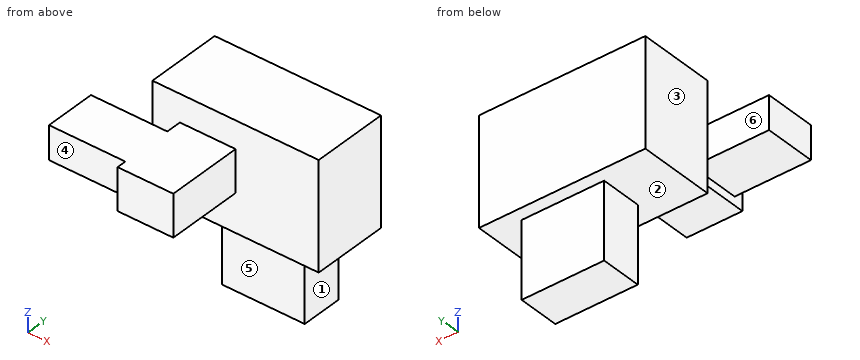
```python
from build123d import *

# Parameters (mm, degrees)
F0_W     = 55.336684
F0_H     = 35.7977
F1_DEPTH = 25.4
F2_W     = 18.540639
F2_H     = 13.976792
F3_DEPTH = 25.4
F4_W     = 17.11444
F4_H     = 11.124386
F5_DEPTH = 25.4
F6_W     = 27.447399
F6_H     = 13.715297
F7_DEPTH = 25.4


with BuildPart() as f1:
    # F0 (on Front) → F1 (new body)
    with BuildSketch(Plane.XZ):
        with Locations((27.668342, 17.89885)):
            Rectangle(F0_W, F0_H)
    extrude(amount=F1_DEPTH)

    # F2 (on face) → F3 (join)
    with BuildSketch(Plane.XZ.offset(25.4)):
        with Locations((18.39802, 19.681605)):
            Rectangle(F2_W, F2_H)
    extrude(amount=F3_DEPTH)

    # F4 (on face) → F5 (join)
    with BuildSketch(Plane(origin=(9.127701, 0, 0), x_dir=(0, -1, 0), z_dir=(-1, 0, 0))):
        with Locations((39.077966, 21.107808)):
            Rectangle(F4_W, F4_H)
    extrude(amount=F5_DEPTH)

    # F6 (on face) → F7 (join)
    with BuildSketch(Plane(origin=(0, 0, 0), x_dir=(1, 0, 0), z_dir=(0, 0, -1))):
        with Locations((30.881432, 11.093259)):
            Rectangle(F6_W, F6_H)
    extrude(amount=F7_DEPTH)


solid = f1.part
```
Build history of the part. All positions in model axes, mm. Face numbers are marked on the shaded views. A direction names the side the tool comes from. Coordinates: 2 decimals unless noted, no trailing zeros. Order: outer loops, then holes, each group sorted by start corner. A loop starts at its lowest first (then second) coordinate and runs counter-clockwise, first axis right, second up. Notation, with made-up numbers: (35, -26) -> (47, -26) arc R16 cw to (47, 4) -> close; hole circle Ø6 at (4, 30). An arc over 180 degrees is marked (long way). Answer in a Markdown table with one row per item. Add a question column.
Q1. Band-saw the part on C-C, the plane z = -7.5. List the corners of the cut face in (x, y).
Q2. Band-saw the part on B-B, the plane y = -40. List the corners of the cut face in (x, z).
Q3. Mould opens along X. For the marked faces 1, 2 and 3 say: +X half, -X half, draft (parallel to the pull), parting line (faces both ways), or undercut.
Q4. Drop flat-ended pins along their axis: pin 1 (5 mm diameter, centred on x = 44.5, z = 20, fed in from -Y); pin 2 (4 mm diameter, centred on y = -10, z = -11.5, fed in from +X); pin 3 (6 mm diameter, centred on x = 26, z = 26.5, fed in from +Y); pin 4 (11 mm diameter, centred on y = -38.5, z = 17.5, fed in from +X). Give the stop position or say it passes through.
Q5. Which spindle directions (+Z, -Z, +X, -X, +Y, -Y) get a long thin tool onto all of the face, cutting with end or side? Do the marked faces 4, 5 and 6. Say none if no direction does.
Q6. Wall check: line 1 along Y through (x, z) = (37.5, 15.5); line 2 along Z through (x, y) = (47.5, -21); line 3 along X through (y, z) = (-2, 27.5). Give the ranges that are in metal, low to high. Write a range as [from, to].
Q7. Band-saw the part on A-A, the plane x = 12. List the corners of the cut face in (y, z), then the cut area to 3 significant figures.
Q8. Band-saw the part on D-D, the plane x = 31.5. List the corners of the cut face in (y, z).
Answers follow:
| question | item | result |
|---|---|---|
| 1 | outline | (17.16, -17.95) -> (44.61, -17.95) -> (44.61, -4.24) -> (17.16, -4.24) -> close |
| 2 | outline | (-16.27, 15.55) -> (9.13, 15.55) -> (9.13, 12.69) -> (27.67, 12.69) -> (27.67, 26.67) -> (-16.27, 26.67) -> close |
| 3 | face 1 | +X half |
| 3 | face 2 | draft |
| 3 | face 3 | -X half |
| 4 | pin 1 | y = -25.4 |
| 4 | pin 2 | x = 44.61 |
| 4 | pin 3 | y = 0 |
| 4 | pin 4 | x = 27.67 |
| 5 | face 4 | +Z, -Z, -X, -Y |
| 5 | face 5 | -Z, +X, -X, -Y |
| 5 | face 6 | +Z, -Z, -X |
| 6 | line 1 | [-25.4, 0] |
| 6 | line 2 | [0, 35.8] |
| 6 | line 3 | [0, 55.34] |
| 7 | outline | (-50.8, 12.69) -> (-25.4, 12.69) -> (-25.4, 0) -> (0, 0) -> (0, 35.8) -> (-25.4, 35.8) -> (-25.4, 26.67) -> (-50.8, 26.67) -> close |
| 7 | area | 1,260 mm^2 |
| 8 | outline | (-25.4, 0) -> (-17.95, 0) -> (-17.95, -25.4) -> (-4.24, -25.4) -> (-4.24, 0) -> (0, 0) -> (0, 35.8) -> (-25.4, 35.8) -> close |
